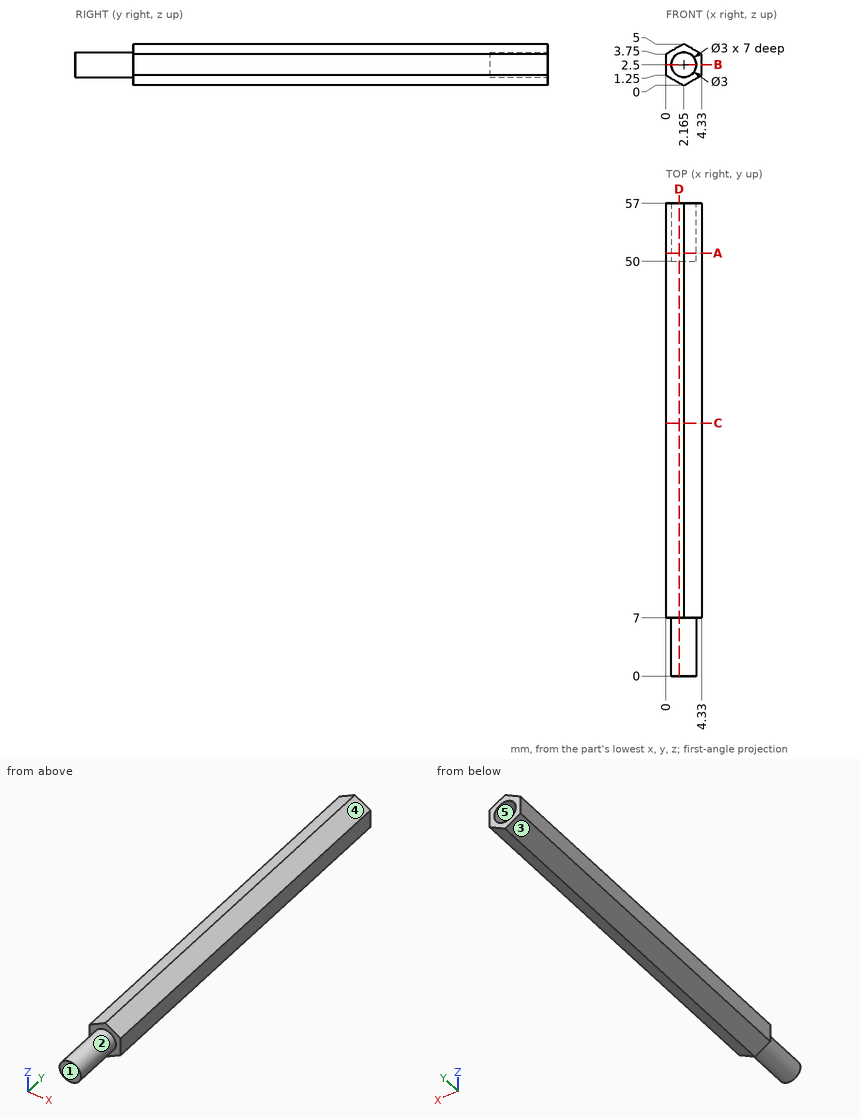
Here's the drawing with two shaded views (mm, measured from the low corner). I have some questions. A direction names the side the tool comes from. Coordinates: 2 decimals unless noted, no trailing zeros. Order: outer loops, then holes, each group sorted by start corner. A loop starts at its lowest first (then second) coordinate and runs counter-clockwise, first axis right, second up.
Item 1: If we section it at D-D, the plane x = 1.6: List the corners of the cut face in (y, z) for me, then the cut area to 3 significant figures.
Response values:
outline: (0, 1.11) - (7, 1.11) - (7, 0.33) - (57, 0.33) - (57, 1.11) - (50, 1.11) - (50, 3.89) - (57, 3.89) - (57, 4.67) - (7, 4.67) - (7, 3.89) - (0, 3.89) - close
area: 217 mm2
Item 2: If we section it at C-C, the plane y = 30.5: List the corners of the cut face in (x, z) for me (3 decimals).
Response values:
outline: (0, 1.25) - (2.165, 0) - (4.33, 1.25) - (4.33, 3.75) - (2.165, 5) - (0, 3.75) - close
Item 3: If we section it at A-A, the plane y = 51: List the corners of the cut face in (x, z) for me (3 decimals).
Response values:
outline: (0, 1.25) - (2.165, 0) - (4.33, 1.25) - (4.33, 3.75) - (2.165, 5) - (0, 3.75) - close; hole circle Ø3 at (2.165, 2.5)
Item 4: I need wall thicknesses on probe 1 along Y at (x, z) = (3.1, 4.15); probe 2 along Z at (x, y) = (3, 2.5); probe 3 along Z at (x, y) = (1.9, 17). Which ranges of each line are inside material? Lowest first, please.
Response values:
probe 1: y = 7 to 57
probe 2: z = 1.25 to 3.75
probe 3: z = 0.15 to 4.85
Item 5: If we section it at B-B, the plane z = 2.5: List the corners of the cut face in (x, y) for me (3 decimals), then the cut area to 4 significant figures.
Response values:
outline: (0, 7) - (0.665, 7) - (0.665, 0) - (3.665, 0) - (3.665, 7) - (4.33, 7) - (4.33, 57) - (3.665, 57) - (3.665, 50) - (0.665, 50) - (0.665, 57) - (0, 57) - close
area: 216.5 mm2
Item 6: Thinking about a two-plate mould opening in X: for the marked faces 3, 4 and 5, which applies, pulls with the +X half, pulls with the -X half, needs draft (parallel to the pull), parting line crosses it, or undercut?
Response values:
face 3: pulls with the -X half
face 4: pulls with the +X half
face 5: undercut
Item 7: I'm going to push a flat-ended pin straight in: pin 1 Ø0.9 at (x, z) = (2.5, 2) entering from +Y. Where does the tip first touch, or does it pass through?
Response values:
pin 1: stops at y = 50
Item 8: Which directions (+Z, -Z, +X, -X, +Y, -Y) give clear straight access to the entire face, cutting with the end or side of a thin tool? Please do the marked faces 1 and 2.
Response values:
face 1: +Z, -Z, +X, -X, -Y
face 2: -Y
